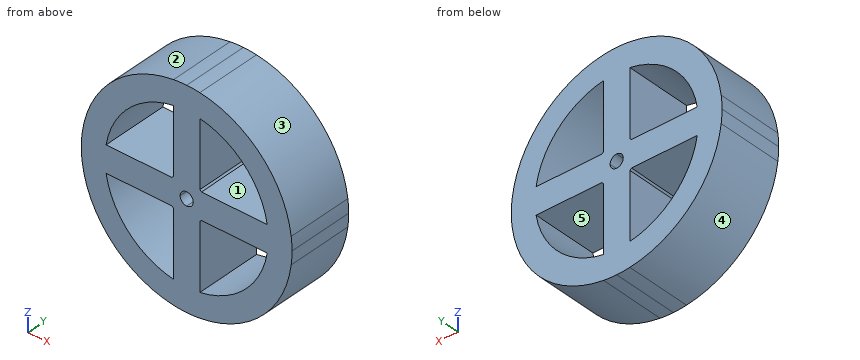
from build123d import *

# Parameters (mm, degrees)
F1_DEPTH = 635


with BuildPart() as f1:
    # F0 (on Front) → F1 (new body)
    with BuildSketch(Plane.XZ):
        with BuildLine():
            Line((0, -1016), (0, -63.5))
            ThreePointArc((0, -63.5), (-44.901281, -44.901281), (-63.5, 0))
            Line((-63.5, 0), (-1016, 0))
            ThreePointArc((-1016, 0), (-1014.005855, -63.624879), (-1008.03125, -127))
            ThreePointArc((-1008.03125, -127), (-718.42049, -718.42049), (-127, -1008.03125))
            ThreePointArc((-127, -1008.03125), (-63.624879, -1014.005855), (0, -1016))
        make_face()
        with BuildLine():
            ThreePointArc((-141.990317, -127), (-134.703842, -134.703842), (-127, -141.990317))
            Line((-127, -141.990317), (-127, -777.090574))
            ThreePointArc((-127, -777.090574), (-556.77588, -556.77588), (-777.090574, -127))
            Line((-777.090574, -127), (-141.990317, -127))
        make_face(mode=Mode.SUBTRACT)
        with BuildLine():
            ThreePointArc((1008.03125, -127), (1014.005855, -63.624879), (1016, 0))
            Line((1016, 0), (63.5, 0))
            ThreePointArc((63.5, 0), (44.901281, -44.901281), (0, -63.5))
            Line((0, -63.5), (0, -1016))
            ThreePointArc((0, -1016), (63.624879, -1014.005855), (127, -1008.03125))
            ThreePointArc((127, -1008.03125), (718.42049, -718.42049), (1008.03125, -127))
        make_face()
        with BuildLine():
            Line((127, -777.090574), (127, -141.990317))
            ThreePointArc((127, -141.990317), (134.703842, -134.703842), (141.990317, -127))
            Line((141.990317, -127), (777.090574, -127))
            ThreePointArc((777.090574, -127), (556.77588, -556.77588), (127, -777.090574))
        make_face(mode=Mode.SUBTRACT)
        with BuildLine():
            ThreePointArc((-63.5, 0), (-44.901281, 44.901281), (0, 63.5))
            Line((0, 63.5), (0, 1016))
            ThreePointArc((0, 1016), (-63.624879, 1014.005855), (-127, 1008.03125))
            ThreePointArc((-127, 1008.03125), (-718.42049, 718.42049), (-1008.03125, 127))
            ThreePointArc((-1008.03125, 127), (-1014.005855, 63.624879), (-1016, 0))
            Line((-1016, 0), (-63.5, 0))
        make_face()
        with BuildLine():
            Line((-127, 777.090574), (-127, 141.990317))
            ThreePointArc((-127, 141.990317), (-134.703842, 134.703842), (-141.990317, 127))
            Line((-141.990317, 127), (-777.090574, 127))
            ThreePointArc((-777.090574, 127), (-556.77588, 556.77588), (-127, 777.090574))
        make_face(mode=Mode.SUBTRACT)
        with BuildLine():
            Line((63.5, 0), (1016, 0))
            ThreePointArc((1016, 0), (1014.005855, 63.624879), (1008.03125, 127))
            ThreePointArc((1008.03125, 127), (718.42049, 718.42049), (127, 1008.03125))
            ThreePointArc((127, 1008.03125), (63.624879, 1014.005855), (0, 1016))
            Line((0, 1016), (0, 63.5))
            ThreePointArc((0, 63.5), (44.901281, 44.901281), (63.5, 0))
        make_face()
        with BuildLine():
            Line((777.090574, 127), (141.990317, 127))
            ThreePointArc((141.990317, 127), (134.703842, 134.703842), (127, 141.990317))
            Line((127, 141.990317), (127, 777.090574))
            ThreePointArc((127, 777.090574), (556.77588, 556.77588), (777.090574, 127))
        make_face(mode=Mode.SUBTRACT)
    extrude(amount=F1_DEPTH)


solid = f1.part
Could you check a few things on this model? Use its own coordinates, in mm. Face numbers are marked on the shaded views. A direction names the side the tool comes from. Coordinates: 2 decimals unless noted, no trailing zeros. Write each loop counter-clockwise with the first axis right and the second up, starting at its lowest first coordinate (ties: lowest second). Pieces come first, ordered by that corner, then holes. Notation, with made-up numbers: (23.5, 57.5) - (42.5, 57.5) arc R31 cw to (42.5, 85.5) - close; hole circle Ø7 at (-29, -27). An arc over 180 degrees is marked (long way). Put each result on its own line as item: value. Start each with the question number.
Q1. Which directions (+Z, -Z, +X, -X, +Y, -Y) give clear straight access to the entire face, cutting with the end or side of a thin tool? Please do the marked faces 4 and 5.
Q2. I want a section at B-B on y = -585. Count the separate pieces of the cut face and the enclosed holes in it, plus the area to 3 significant figures.
Q3. I want a section at C-C on z = -472. Write out the boundary of the cut face in (x, y).
Q4. Please list where these lines run through material, in increasing order: L1, parallel to Z at x = 506, y = -62.5; L2, parallel to Z at x = -130.5, y = -71.5; L3, parallel to X at y = -562, z = -324.
Q5. I want a section at A-A on x = -315. Write out the boundary of the cut face in (y, z).
Q6. Thinking about a two-plate mould opening in X: for the marked faces 1, 2 and 3, which applies, pulls with the +X half, pulls with the -X half, needs draft (parallel to the pull), parting line crosses it, or undercut?
Q7. I'm going to push flat-ended pins straight in: P1, Ø3, axis at x = -665, y = -503, coming from the +Z side; P2, Ø8, axis at y = -120.5, z = -238, coming from the -X side; P3, Ø3, axis at y = -90, z = 742.5, coming from the -X side; P4, Ø1, axis at x = -609, z = -128.5, coming from the +Y side. Where does each tip first touch, or does it pass through?
Checks:
1. face 4: -Z, -X, +Y, -Y
1. face 5: +Y, -Y
2. separate pieces: 1
2. enclosed holes: 5
2. area: 2,010,000 mm²
3. outline: (-899.71, -635) - (-630.25, -635) - (-630.25, 0) - (-899.71, 0) - close; (-127, -635) - (127, -635) - (127, 0) - (-127, 0) - close; (630.25, -635) - (899.71, -635) - (899.71, 0) - (630.25, 0) - close
4. L1: -881.03 to -603.29, -127 to 127, 603.29 to 881.03
4. L2: -1007.58 to -776.51, -138.78 to 138.78, 776.51 to 1007.58
4. L3: -962.95 to -717.65, -127 to 127, 717.65 to 962.95
5. outline: (-635, -965.94) - (0, -965.94) - (0, -721.65) - (-635, -721.65) - close; (-635, -127) - (0, -127) - (0, 127) - (-635, 127) - close; (-635, 721.65) - (0, 721.65) - (0, 965.94) - (-635, 965.94) - close
6. face 1: undercut
6. face 2: pulls with the -X half
6. face 3: pulls with the +X half
7. P1: z = 769.43
7. P2: x = -988.69
7. P3: x = -695.11
7. P4: through
